from build123d import *

# Parameters (mm, degrees)
SKETCH1_R           = 20.5
BOSS_EXTRUDE1_DEPTH = 7
SKETCH2_R           = 2.675
CUT_EXTRUDE1_DEPTH  = 7
BOSS_EXTRUDE2_START = 0.4
SKETCH3_R           = 3.425
SKETCH3_R_2         = 2.675
BOSS_EXTRUDE2_DEPTH = 0.4
CUT_EXTRUDE3_DEPTH  = 7


with BuildPart() as part:
    # Sketch1 → Boss-Extrude1 (new body)
    with BuildSketch(Plane(origin=(0, 0, 0), x_dir=(1, 0, 0), z_dir=(0, 1, 0))):
        with Locations(Location((0, 0, 0), (0, 0, 270))):
            Circle(SKETCH1_R)
    extrude(amount=BOSS_EXTRUDE1_DEPTH)

    # Sketch2 → Cut-Extrude1 (cut)
    with BuildSketch(Plane(origin=(0, 7, 0), x_dir=(1, 0, 0), z_dir=(0, 1, 0))):
        with Locations(Location((0, 0, 0), (0, 0, 270))):
            Circle(SKETCH2_R)
    extrude(amount=-CUT_EXTRUDE1_DEPTH, mode=Mode.SUBTRACT)

    # Sketch3 → Boss-Extrude2 (add)
    with BuildSketch(Plane(origin=(0, 7, 0), x_dir=(1, 0, 0), z_dir=(0, 1, 0)).offset(BOSS_EXTRUDE2_START)):
        with Locations(Location((0, 0, 0), (0, 0, 270))):
            Circle(SKETCH3_R)
        with Locations(Location((0, 0, 0), (0, 0, 270))):
            Circle(SKETCH3_R_2, mode=Mode.SUBTRACT)
    extrude(amount=-BOSS_EXTRUDE2_DEPTH)

    # Sketch5 → Cut-Extrude3 (cut)
    with BuildSketch(Plane(origin=(0, 7, 0), x_dir=(1, 0, 0), z_dir=(0, 1, 0))):
        with BuildLine():
            Line((-6, 15), (6, 15))
            ThreePointArc((6, 15), (11, 10), (6, 5))
            Line((6, 5), (-6, 5))
            ThreePointArc((-6, 5), (-11, 10), (-6, 15))
        make_face()
    extrude(amount=-CUT_EXTRUDE3_DEPTH, mode=Mode.SUBTRACT)


solid = part.part
Design review of the part built by this model. Coordinates are the model's own, in mm. A direction names the side the tool comes from. Coordinates: 2 decimals unless noted, no trailing zeros. Order: outer loops, then holes, each group sorted by start corner. A loop starts at its lowest first (then second) coordinate and runs counter-clockwise, first axis right, second up. Notation, with made-up numbers: (13, -1.75) -> (22, -1.75) arc R29 cw to (22, 20.25) -> close; hole circle Ø3 at (-23.75, 33). An arc over 180 degrees is marked (long way). One line per item, written item: value.
1) To check wall thickness, follow probe 1 along X at (y, z) = (4.25, 0) (3 decimals); probe 2 along Z at (x, y) = (1, 2.25); probe 3 along Y at (x, z) = (-15.5, -1.5). State the ranges of each line that lie inside material, in increasing order. Write a range as [from, to].
Output values:
probe 1: x = [-20.5, -2.675], [2.675, 20.5]
probe 2: z = [-20.48, -15], [-5, -2.48], [2.48, 20.48]
probe 3: y = [0, 7]
2) Clearance check with flat-ended pins moving along their axes: P1, Ø4, axis at x = -4, y = 3, coming from the +Z side; P2, Ø1, axis at y = 2, z = 6.5, coming from the +X side; P3, Ø1.5, axis at y = 1, z = 12.5, coming from the -X side. State where each tip first meets the part, or that it passes through.
Output values:
P1: stops at z = 20.4
P2: stops at x = 19.6
P3: stops at x = -16.8
3) Machinability: for faces 5 (the face through (1.029, 7.203, 3.267)), 6 (the face through (0, 4, -15)), 7 (the face through (0, 0, 4)), which of the approach directions +Z, -Z, +X, -X, +Y, -Y give a long, thin tool a straight path to every point of the face, cutting with its end or side? Answer none if there is none.
Output values:
face 5: +Y
face 6: +Y, -Y
face 7: +Z, -Z, +X, -X, -Y
4) We need section D-D, the plane z = -7.5. Give the boundary of the cut face in (x, y), then the cut area to 3 significant figures.
Output values:
outline: (-19.08, 0) -> (-10.33, 0) -> (-10.33, 7) -> (-19.08, 7) -> close; (10.33, 0) -> (19.08, 0) -> (19.08, 7) -> (10.33, 7) -> close
area: 122 mm2
5) We need section A-A, the plane z = 0. Give the boundary of the cut face in (x, y) (3 decimals), then the cut area to 3 significant figures.
Output values:
outline: (-20.5, 0) -> (-2.675, 0) -> (-2.675, 7.4) -> (-3.425, 7.4) -> (-3.425, 7) -> (-20.5, 7) -> close; (2.675, 0) -> (20.5, 0) -> (20.5, 7) -> (3.425, 7) -> (3.425, 7.4) -> (2.675, 7.4) -> close
area: 250 mm2
6) Draft analysis for pull direction X (two halves, no side actions). For faces 1 (the face through (-20.013, 3.451, -4.444)), 2 (the face through (0, 4, -5)), 3 (the face through (0, 7, 4)), 4 (the face through (-11, 4, -10)), state which applies: +X half, -X half, draft (parallel to the pull), parting line (faces both ways), or undercut.
Output values:
face 1: parting line
face 2: undercut
face 3: draft
face 4: undercut
7) We need section C-C, the plane y = 1. Give the boundary of the cut face in (x, z) (3 decimals).
Output values:
outline: circle Ø41 at (0, 0); hole (-6, -15) -> (6, -15) arc R5 ccw to (6, -5) -> (-6, -5) arc R5 ccw to start; hole circle Ø5.35 at (0, 0)
8) We need section B-B, the plane x = 6.5. Give the boundary of the cut face in (y, z), then the cut area to 3 significant figures.
Output values:
outline: (0, -19.44) -> (7, -19.44) -> (7, -14.97) -> (0, -14.97) -> close; (0, -5.03) -> (7, -5.03) -> (7, 19.44) -> (0, 19.44) -> close
area: 203 mm2
